Autodesk Inventor part; units mm, degrees
ref_plane "YZ Plane" through (0, 0, 0) normal (1, 0, 0) x (0, 1, 0)
ref_plane "XZ Plane" through (0, 0, 0) normal (0, 1, 0) x (-1, 0, 0)
ref_plane "XY Plane" through (0, 0, 0) normal (0, 0, 1) x (1, 0, 0)
sketch "スケッチ1" plane through (0, 0, 0) normal (0, 0, 1) x (1, 0, 0)
  line L0 (-5.05, 5.05) -> (5.05, 5.05)
  line L1 (5.05, 5.05) -> (5.05, -5.05)
  line L2 (5.05, -5.05) -> (-5.05, -5.05)
  line L3 (-5.05, -5.05) -> (-5.05, 5.05)
  line L4 (0, -9.87) -> (0, 9.87)
  line L5 (-9.87, 0) -> (9.87, 0)
  line L6 (7.05, 7.05) -> (-7.05, 7.05)
  line L7 (-7.05, 7.05) -> (-7.05, -7.05)
  line L8 (-7.05, -7.05) -> (7.05, -7.05)
  line L9 (7.05, -7.05) -> (7.05, 7.05)
  point P0 (0, 0)
  dimension "d0" = 10.1
  dimension "d1" = 2
  dimension "d27" = 10.1
extrude "押し出し1" add sketch "スケッチ1" along normal mid plane 10.1 contours L3 L5 L7 L6 L4 L0 | L4 L6 L9 L5 L1 L0 | L3 L2 L4 L8 L7 L5 | L5 L9 L8 L4 L2 L1
sketch "スケッチ2" plane through (0, 0, -5.05) normal (0, 0, -1) x (-1, 0, 0)
  line L0 (-7.05, -7.05) -> (-7.05, 7.05)
  line L1 (7.05, 7.05) -> (-7.05, 7.05)
  line L2 (-7.05, -7.05) -> (7.05, -7.05)
  line L3 (7.05, -7.05) -> (7.05, 7.05)
  line L4 (7.05, 7.05) -> (-7.05, 7.05)
  line L5 (-7.05, 7.05) -> (-7.05, -7.05)
  line L6 (5.05, 5.05) -> (5.05, -5.05)
  line L7 (5.05, -5.05) -> (-5.05, -5.05)
  line L8 (-5.05, -5.05) -> (-5.05, 5.05)
  line L9 (-5.05, 5.05) -> (5.05, 5.05)
  line L10 (-7.05, 7.05) -> (7.05, 7.05)
  line L11 (-7.05, 7.05) -> (7.05, 7.05)
  line L12 (7.05, 7.05) -> (7.05, -7.05)
  line L13 (7.05, -7.05) -> (-7.05, -7.05)
  line L14 (9.87, 0) -> (-9.87, 0)
  line L15 (0, -10.0068) -> (0, 10.0068)
  line L16 (-7.05, 7.05) -> (-7.05, -7.05)
  line L17 (7.05, 7.05) -> (7.05, -7.05)
  point P0 (0, 0)
extrude "押し出し2" add sketch "スケッチ2" along normal blind 3
sketch "スケッチ4" plane through (0, 0, -8.05) normal (0, 0, -1) x (-1, 0, 0)
  line L0 (3.5, 1.5) -> (-3.5, 1.5)
  line L1 (-3.5, 1.5) -> (-3.5, -1.5)
  line L2 (-3.5, -1.5) -> (3.5, -1.5)
  line L3 (3.5, -1.5) -> (3.5, 1.5)
  line L4 (9.87, 0) -> (-9.87, 0)
  line L5 (0, -9.87) -> (0, 9.87)
  point P0 (0, 0)
  dimension "d19" = 3
  dimension "d20" = 7
extrude "押し出し4" add sketch "スケッチ4" along normal blind 11
sketch "スケッチ5" plane through (-3.5, 1.5, -8.05) normal (0, 1, 0) x (1, 0, 0)
  circle A0 centre (3.5, 6.5) radius 1.5
  line L0 (-3.55, 0) -> (10.55, 0)
  line L1 (3.5, 15.82) -> (3.5, -17.92)
  point P0 (3.5, -8.05)
  dimension "d23" = 3
  dimension "d24" = 6.5
extrude "押し出し5" cut sketch "スケッチ5" against normal up to surface (3 mm away)
properties part number "adapter_for_magnet"
Work out the finished part from the listing and answer in its coordinate system (mm). A direction names the side the tool comes from. Give positions to 0.01 mm unless a question says otherwise; leave off trailing zeros. Write each loop counter-clockwise with the first axis right and the second up, starting at its lowest first coordinate (ties: lowest second). Pieces come first, ordered by that corner, then holes. Notation, with made-up numbers: (2, 72.5) -> (45, 72.5) arc R33 cw to (45, 103.5) -> close; hole circle Ø4 at (65.5, -6). An arc over 180 degrees is marked (long way). Write each question's results on one line, items separated by ' | '.
1. Find section D-D on z = 2.5. Determine the outline of the cut face in (x, y), and give its area (3 significant figures).
Data:
outline: (-7.05, -7.05) -> (7.05, -7.05) -> (7.05, 7.05) -> (-7.05, 7.05) -> close; hole (-5.05, -5.05) -> (5.05, -5.05) -> (5.05, 5.05) -> (-5.05, 5.05) -> close | area: 96.8 mm^2
2. A tool of negligible diameter and unlimited length cuts with its end or side. For faces 4 (the flat face through (0, 1.5, -12)), 5 (the flat face through (-3.5, 0, -13)), 6 (the flat face through (5.05, 0, 0)), 7 (the flat face through (-7.05, 0, -2)), from which of +Z, -Z, +X, -X, +Y, -Y can it reach the whole face along a straight path? Write none if from no direction.
Data:
face 4: -Z, +X, -X, +Y | face 5: -Z, -X, +Y, -Y | face 6: +Z | face 7: +Z, -Z, -X, +Y, -Y
3. Find section B-B on x = 0. Determine the outline of the cut face in (y, z), and give its area (3 significant figures).
Data:
outline: (-7.05, -8.05) -> (-1.5, -8.05) -> (-1.5, -13.05) -> (1.5, -13.05) -> (1.5, -8.05) -> (7.05, -8.05) -> (7.05, 5.05) -> (5.05, 5.05) -> (5.05, -5.05) -> (-5.05, -5.05) -> (-5.05, 5.05) -> (-7.05, 5.05) -> close; (-1.5, -19.05) -> (1.5, -19.05) -> (1.5, -16.05) -> (-1.5, -16.05) -> close | area: 107 mm^2
4. Determine the mould class of faces 1 (the flat face through (0, -1.5, -12)), 2 (the flat face through (0, 0, -5.05)), 3 (the flat face through (3.5, 0, -13)) for opening direction Y: +Y half, -Y half, draft (parallel to the pull), parting line (faces both ways), or undercut.
Data:
face 1: -Y half | face 2: undercut | face 3: draft
5. Find section A-A on z = -14.55. Determine the outline of the cut face in (x, y).
Data:
outline: (-3.5, -1.5) -> (-1.5, -1.5) -> (-1.5, 1.5) -> (-3.5, 1.5) -> close; (1.5, -1.5) -> (3.5, -1.5) -> (3.5, 1.5) -> (1.5, 1.5) -> close
6. Straight lines are drawn through the part: L1, parallel to X at y = -0.65, z = -14.55; L2, parallel to Z at x = 0, y = -0.6; L3, parallel to Y at x = -1.25, z = -2.25. For each, find the intervals that lie inside material, in ascending order.
Data:
L1: -3.5 to -1.5, 1.5 to 3.5 | L2: -19.05 to -16.05, -13.05 to -5.05 | L3: -7.05 to -5.05, 5.05 to 7.05
7. Find section C-C on y = -0.25. Determine the outline of the cut face in (x, z), and give its area (3 significant figures).
Data:
outline: (-7.05, -8.05) -> (-3.5, -8.05) -> (-3.5, -19.05) -> (3.5, -19.05) -> (3.5, -8.05) -> (7.05, -8.05) -> (7.05, 5.05) -> (5.05, 5.05) -> (5.05, -5.05) -> (-5.05, -5.05) -> (-5.05, 5.05) -> (-7.05, 5.05) -> close; hole circle Ø3 at (0, -14.55) | area: 153 mm^2
8. Each of these flat-tipped pins is pushed along its axis until it touches: pin 1 Ø2 at (x, y) = (-3.5, -3) entering from -Z; pin 2 Ø4 at (x, z) = (-1.5, -16) entering from -Y; pin 3 Ø3 at (y, z) = (-0.5, -16) entering from +X. Where does it stop, or does it pass through?
Data:
pin 1: z = -8.05 | pin 2: y = -1.5 | pin 3: x = 3.5
